from build123d import *

# Parameters (mm, degrees)
SALIENTE_EXTRUIR1_DEPTH = 105
CROQUIS3_W              = 4
CROQUIS3_H              = 30
SALIENTE_EXTRUIR2_DEPTH = 30
CROQUIS4_W              = 77
CROQUIS4_H              = 30
CORTAR_EXTRUIR1_DEPTH   = 30
CROQUIS5_W              = 81
CROQUIS5_H              = 50
CORTAR_EXTRUIR2_DEPTH   = 30
CROQUIS6_W              = 4
CROQUIS6_H              = 30
CORTAR_EXTRUIR3_DEPTH   = 70
SALIENTE_EXTRUIR4_DEPTH = 40
CROQUIS7_W              = 30
CROQUIS7_H              = 6
SALIENTE_EXTRUIR5_DEPTH = 4
CROQUIS10_W             = 5
CROQUIS10_H             = 40
CORTAR_EXTRUIR5_DEPTH   = 4
CROQUIS11_W             = 10
CROQUIS11_H             = 40
CORTAR_EXTRUIR6_DEPTH   = 4
CROQUIS12_R             = 2.5
CORTAR_EXTRUIR7_DEPTH   = 90
CROQUIS13_W             = 5
CROQUIS13_H             = 40
CORTAR_EXTRUIR8_DEPTH   = 10


with BuildPart() as part:
    # Croquis2 → Saliente-Extruir1 (new body)
    with BuildSketch(Plane.XY):
        Polygon((47.018573694, 40), (43.018573694, 40), (43.018573694, 4), (-37.981426306, 4), (-37.981426306, 40), (-41.981426306, 40), (-41.981426306, 0), (47.018573694, 0), align=None)
    extrude(amount=SALIENTE_EXTRUIR1_DEPTH)

    # Croquis3 → Saliente-Extruir2 (add)
    with BuildSketch(Plane.XY):
        with Locations((-35.981426306, 25)):
            Rectangle(CROQUIS3_W, CROQUIS3_H)
    extrude(amount=SALIENTE_EXTRUIR2_DEPTH)

    # Croquis4 → Cortar-Extruir1 (cut)
    with BuildSketch(Plane(origin=(0, 4, 0), x_dir=(1, 0, 0), z_dir=(0, 1, 0))):
        with Locations((4.518573694, -15)):
            Rectangle(CROQUIS4_W, CROQUIS4_H)
    extrude(amount=-CORTAR_EXTRUIR1_DEPTH, mode=Mode.SUBTRACT)

    # Croquis5 → Cortar-Extruir2 (cut)
    with BuildSketch(Plane(origin=(0, 4, 0), x_dir=(1, 0, 0), z_dir=(0, 1, 0))):
        with Locations((2.518573694, -80)):
            Rectangle(CROQUIS5_W, CROQUIS5_H)
    extrude(amount=-CORTAR_EXTRUIR2_DEPTH, mode=Mode.SUBTRACT)

    # Croquis6 → Cortar-Extruir3 (cut)
    with BuildSketch(Plane(origin=(0, 40, 0), x_dir=(1, 0, 0), z_dir=(0, 1, 0))):
        with Locations((-39.981426306, -15)):
            Rectangle(CROQUIS6_W, CROQUIS6_H)
        Polygon((-41.981426306, -30), (-41.981426306, -35), (-37.981426306, -30), align=None)
    extrude(amount=-CORTAR_EXTRUIR3_DEPTH, mode=Mode.SUBTRACT)

    # Croquis8 → Saliente-Extruir4 (add)
    with BuildSketch(Plane(origin=(0, 40, 0), x_dir=(1, 0, 0), z_dir=(0, 1, 0))):
        Polygon((-37.981426306, -30), (-33.981426306, -30), (-37.981426306, -35), align=None)
    extrude(amount=-SALIENTE_EXTRUIR4_DEPTH)

    # Croquis7 → Saliente-Extruir5 (add)
    with BuildSketch(Plane.ZY.offset(37.981426306)):
        with Locations((15, 7)):
            Rectangle(CROQUIS7_W, CROQUIS7_H)
    extrude(amount=-SALIENTE_EXTRUIR5_DEPTH)

    # Croquis10 → Cortar-Extruir5 (cut)
    with BuildSketch(Plane(origin=(47.018573694, 0, 0), x_dir=(0, 0, -1), z_dir=(1, 0, 0))):
        with Locations((-2.5, 20)):
            Rectangle(CROQUIS10_W, CROQUIS10_H)
    extrude(amount=-CORTAR_EXTRUIR5_DEPTH, mode=Mode.SUBTRACT)

    # Croquis11 → Cortar-Extruir6 (cut)
    with BuildSketch(Plane(origin=(47.018573694, 0, 0), x_dir=(0, 0, -1), z_dir=(1, 0, 0))):
        with Locations((-100, 20)):
            Rectangle(CROQUIS11_W, CROQUIS11_H)
    extrude(amount=-CORTAR_EXTRUIR6_DEPTH, mode=Mode.SUBTRACT)

    # Croquis12 → Cortar-Extruir7 (cut, through all)
    with BuildSketch(Plane(origin=(47.018573694, 0, 0), x_dir=(0, 0, -1), z_dir=(1, 0, 0))):
        with Locations((-15, 20)):
            Circle(CROQUIS12_R)
        with Locations((-85, 20)):
            Circle(CROQUIS12_R)
    extrude(amount=-CORTAR_EXTRUIR7_DEPTH, mode=Mode.SUBTRACT)

    # Croquis13 → Cortar-Extruir8 (cut)
    with BuildSketch(Plane.ZY.offset(37.981426306)):
        with Locations((2.5, 20)):
            Rectangle(CROQUIS13_W, CROQUIS13_H)
    extrude(amount=-CORTAR_EXTRUIR8_DEPTH, mode=Mode.SUBTRACT)


solid = part.part
Model file for the job. Use its own axes, mm. A direction names the side the tool comes from. Give positions to 0.01 mm unless a question says otherwise; leave off trailing zeros. Order: outer loops, then holes, each group sorted by start corner. A loop starts at its lowest first (then second) coordinate and runs counter-clockwise, first axis right, second up. Notation, with made-up numbers: (48, 45.5) - (72, 45.5) arc R21 ccw to (72, 67.5) - close; hole circle Ø5 at (-21.5, -22). An arc over 180 degrees is marked (long way). One line per item, written item: value.
Item 1: Slice it at B-B (z = 85). List the corners of the cut face in (x, y), then the cut area to 3 significant figures.
Response values:
outline: (-41.98, 0) - (-37.98, 0) - (-37.98, 17.5) - (-41.98, 17.5) - close; (-41.98, 22.5) - (-37.98, 22.5) - (-37.98, 40) - (-41.98, 40) - close; (43.02, 0) - (47.02, 0) - (47.02, 17.5) - (43.02, 17.5) - close; (43.02, 22.5) - (47.02, 22.5) - (47.02, 40) - (43.02, 40) - close
area: 280 mm2
Item 2: Slice it at A-A (y = 35). List the corners of the cut face in (x, z), then the cut area to 3 significant figures.
Response values:
outline: (-41.98, 35) - (-37.98, 30) - (-37.98, 5) - (-33.98, 5) - (-33.98, 30) - (-37.98, 35) - (-37.98, 105) - (-41.98, 105) - close; (43.02, 5) - (47.02, 5) - (47.02, 95) - (43.02, 95) - close
area: 760 mm2
Item 3: Wall check: line 1 (X direction, y = 32.5, z = 57); line 2 (Y direction, x = 45.65, z = 15); line 3 (X direction, y = 29, z = 20). Give the ranges that are in metal, low to high.
Response values:
line 1: -41.98 to -37.98, 43.02 to 47.02
line 2: 0 to 17.5, 22.5 to 40
line 3: -37.98 to -33.98, 43.02 to 47.02
Item 4: Two-plate mould, pull along X, no slides. Class faces 1 (the flat face through (2, 2, 55)), 2 (the flat face through (-40, 20, 105)), 3 (the flat face through (47.019, 20, 49)): released by +X, released by -X, zero draft, split by the parting line, or undercut.
Response values:
face 1: undercut
face 2: zero draft
face 3: released by +X
Item 5: Tool access for faces 4 (the flat face through (-35.953, 22.252, 32.465)), 5 (the flat face through (45, 20, 95)), 6 (the flat face through (-39, 40, 54)), 7 (the flat face through (4, 2, 30)), 8 (the flat face through (-37.981, 20, 20)): list every direction of +Z, -Z, +X, -X, +Y, -Y with a clear straight run to the whole face (end or side of a thin tool).
Response values:
face 4: +Z, +Y
face 5: +Z, +X, +Y, -Y
face 6: +Z, -Z, +X, -X, +Y
face 7: -Z, +Y, -Y
face 8: -Z, -X, +Y, -Y
Item 6: Slice it at C-C (z = 11). List the corners of the cut face in (x, y), then the cut area to 3 significant figures.
Response values:
outline: (-37.98, 0) - (-33.98, 0) - (-33.98, 40) - (-37.98, 40) - close; (43.02, 0) - (47.02, 0) - (47.02, 40) - (43.02, 40) - close
area: 320 mm2
Item 7: Pin check, flat tips, straight feed: pin 1 Ø6 at (y, z) = (20, 15) entering from -X; pin 2 Ø1.2 at (x, y) = (2, 1) entering from -Z; pin 3 Ø10 at (x, y) = (-14.5, 7) entering from +Z; pin 4 Ø4.5 at (y, z) = (20, 85) entering from -X. Stop position of each tip, or through.
Response values:
pin 1: x = -37.98
pin 2: z = 30
pin 3: z = 55
pin 4: through
Item 8: Slice it at D-D (x = 33). List the corners of the cut face in (y, z).
Response values:
outline: (0, 30) - (4, 30) - (4, 55) - (0, 55) - close
